The figure shows three views and two pictorial views of one solid part (mm, origin at its lowest corner). Answer the questions. Round coordinates to 2 decimals unless told otherwise and drop trailing zeros. Order: outer loops, then holes, each group sorted by start corner. A loop starts at its lowest first (then second) coordinate and runs counter-clockwise, first axis right, second up. Notation, with made-up numbers: M 38,87 L 47,87 A13 ccw 47,97 Z; hole C 29.5,0 d5. An arc over 180 degrees is marked long. Return JSON: item names as keys, results as strings.
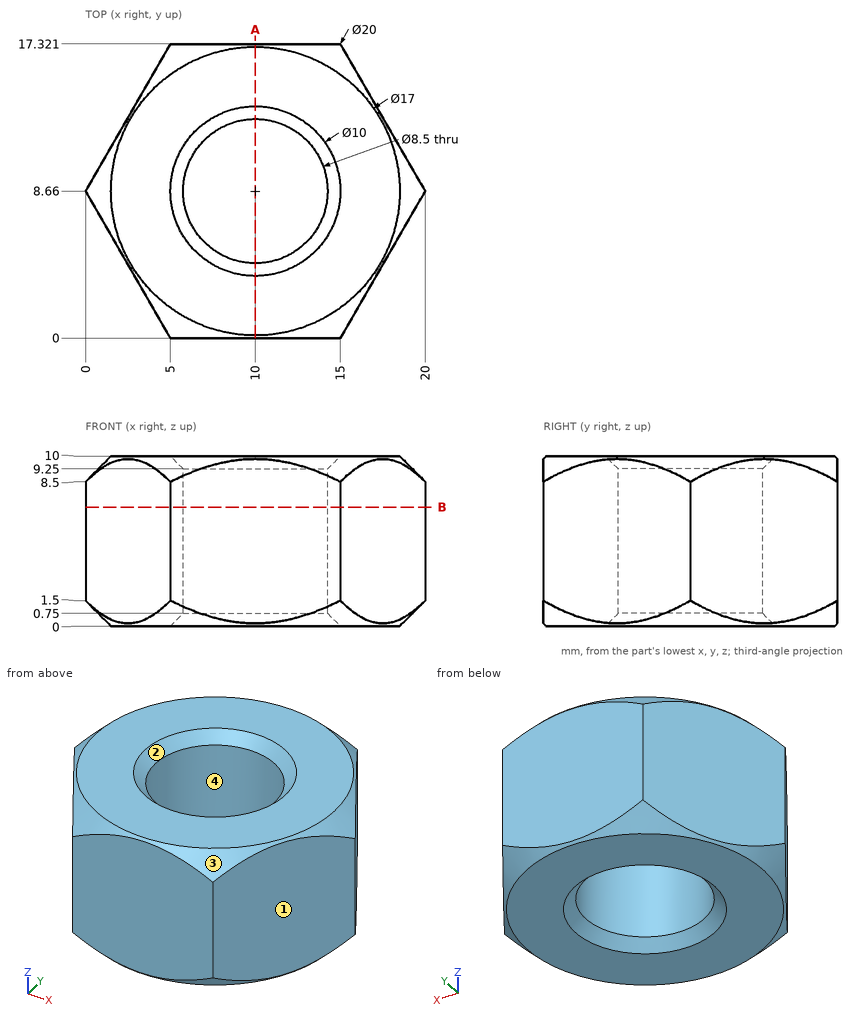
Item 1: The mould has two halves that part along X. Classify the marked faces 1, 2, 3 and 4: pulls with the +X half, pulls with the -X half, needs draft (parallel to the pull), parting line crosses it, or undercut.
Output:
{"face 1": "pulls with the +X half", "face 2": "undercut", "face 3": "parting line crosses it", "face 4": "undercut"}
Item 2: Find section A-A (x = 10). Determine the outline of the cut face in (y, z).
Output:
{"outline": "M 0,0.16 L 0.16,0 L 3.66,0 L 4.41,0.75 L 4.41,9.25 L 3.66,10 L 0.16,10 L 0,9.84 Z; M 12.91,0.75 L 13.66,0 L 17.16,0 L 17.32,0.16 L 17.32,9.84 L 17.16,10 L 13.66,10 L 12.91,9.25 Z"}
Item 3: Consider line 1 along Y through (x, z) = (10, 6.25); line 2 along X through (y, z) = (5.5, 6) (1 decimal); line 3 along X through (y, z) = (5, 3.75) (1 decimal). Determine where each line is inside the solid, lowest interval first. Write a range as [from, to].
Output:
{"line 1": "y = [0, 4.41], [12.91, 17.32]", "line 2": "x = [1.8, 7.2], [12.8, 18.2]", "line 3": "x = [2.1, 7.8], [12.2, 17.9]"}
Item 4: Each of these flat-tipped pins is pushed along its axis until it touches: pin 1 (2 mm diameter, centred on y = 4.5, z = 3.5, fed in from -X) (1 decimal); pin 2 (1.5 mm diameter, centred on x = 3, z = 6.5, fed in from -Y) (1 decimal); pin 3 (2 mm diameter, centred on y = 3.5, z = 7.5, fed in from +X). Where does it stop, or does it pass through?
Output:
{"pin 1": "stops at x = 1.8", "pin 2": "stops at y = 2.2", "pin 3": "stops at x = 17.6"}
Item 5: Find section B-B (z = 7). Determine the outline of the cut face in (x, y), plus the area to 3 significant figures.
Output:
{"outline": "M 0,8.66 L 5,0 L 15,0 L 20,8.66 L 15,17.32 L 5,17.32 Z; hole C 10,8.66 d8.5", "area": "203 mm^2"}
